Design review of the part built by this model. Coordinates are the model's own, in mm. A direction names the side the tool comes from. Give positions to 0.01 mm unless a question says otherwise; leave off trailing zeros. Write each loop counter-clockwise with the first axis right and the second up, starting at its lowest first coordinate (ties: lowest second). Pieces come first, ordered by that corner, then holes. Notation, with made-up numbers: M -11.75,73 L -3.75,73 A16 cw -3.75,89 Z; hole C 7,74.25 d4. An arc over 180 degrees is marked long. Write each question's results on one line, items separated by ' | '. Start each with the question number.
Autodesk Inventor part; units mm, degrees
ref_plane "YZ Plane" through (0, 0, 0) normal (1, 0, 0) x (0, 1, 0)
ref_plane "XZ Plane" through (0, 0, 0) normal (0, 1, 0) x (-1, 0, 0)
ref_plane "XY Plane" through (0, 0, 0) normal (0, 0, 1) x (1, 0, 0)
sketch "Sketch1" plane through (0, 0, 0) normal (0, 0, 1) x (1, 0, 0)
  arc A0 (25.4346, -0.9988) -> (-25.4346, 0.9988) centre (0, 0) ccw
  arc A1 (-58.3107, -836.2235) -> (-7.4415, -838.2211) centre (-32.8761, -837.2223) ccw
  arc A2 (-63.0695, -836.0367) -> (-2.6827, -838.4079) centre (-32.8761, -837.2223) ccw
  arc A3 (30.1934, -1.1856) -> (-30.1934, 1.1856) centre (0, 0) ccw
  line L0 (-30.1934, 1.1856) -> (-63.0695, -836.0367)
  line L1 (-58.3107, -836.2235) -> (-25.4346, 0.9988)
  line L2 (25.4346, -0.9988) -> (-7.4415, -838.2211)
  line L3 (-2.6827, -838.4079) -> (30.1934, -1.1856)
  dimension "d0" = 4.7625
extrude "Extrusion1" add sketch "Sketch1" along normal blind 4.7625
fillet "Fillet1" radius 2.3813 8 edges at (-34.0618, -867.4157, 4.7625) (-46.6315, -417.4255, 4.7625) (1.1856, 30.1934, 4.7625) (13.7554, -419.7968, 4.7625) (1.1856, 30.1934, 0) (-46.6315, -417.4255, 0) (-34.0618, -867.4157, 0) (13.7554, -419.7968, 0)
properties part number "Belt_Vertical_Long2"
Q1. For faces 3 (the flat face through (9.227, -413.749, 2.348)), 4 (the cylindrical face through (13.31, -413.91, 0.72)), list the 3-axis set-ups (+Z, -Z, +X, -X, +Y, -Y) from which the entire face can be reached by the end or side of a thin tool; tool diameter is ignored.
Q2. We need section A-A on z = 1.25. Write out the cut boundary in (x, y), and give its area (3 significant figures).
Q3. The part is to be moulded in two halves that separate along Y. For faces 1 (the cylindrical face through (0.44, 25.45, 2.35)), 2 (the flat face through (10, -417, 4.762)), say which applies: pulls with the +Y half, pulls with the -Y half, needs draft (parallel to the pull), parting line crosses it, or undercut.
Q4. For pin 1 Ø2 at (x, z) = (-24.5, 2) entering from -Y; pin 2 Ø1.5 at (y, z) = (-526.5, 1.5) entering from +X; pin 3 Ø2 at (y, z) = (-361, 1.5) entering from +X, all flat-tipped, find the tip position at first contact; note any pin that passes through.
Q5. Wall thickness on line 1 along X through (y, z) = (-282, 1.75); line 2 along X through (y, z) = (-772, 2.75); line 3 along Y through (x, z) = (-15, 3.6): over which ranges is each line inside the solid? List them lowest first. Write a range as from..to.
Answer sheet:
1) face 3: +Z, -Z | face 4: -Z, +X, -Y
2) outline: M -62.78,-836.05 A29.93 ccw -2.97,-838.4 L 29.91,-1.17 A29.93 ccw -29.91,1.17 Z; hole M -58.31,-836.22 A25.45 ccw -7.44,-838.22 L 25.43,-1 A25.45 ccw -25.43,1 Z | area: 8,280 mm^2
3) face 1: undercut | face 2: needs draft
4) pin 1: y = -866.51 | pin 2: x = 9.57 | pin 3: x = 16.09
5) line 1: -41.23..-36.55, 14.4..19.08 | line 2: -60.53..-55.79, -4.84..-0.1 | line 3: -861.17..-855.34, 20.56..25.84
